from build123d import *

# Parameters (mm, degrees)
SKETCH1_R           = 45
SKETCH1_R_2         = 15
SKETCH1_R_3         = 2.5
BOSS_EXTRUDE1_DEPTH = 3
SKETCH2_R           = 4
SKETCH2_R_2         = 2.5
BOSS_EXTRUDE2_DEPTH = 1
FILLET1_R           = 0.25


with BuildPart() as part:
    # Sketch1 → Boss-Extrude1 (new body)
    with BuildSketch(Plane(origin=(0, 0, 0), x_dir=(1, 0, 0), z_dir=(0, 1, 0))):
        with Locations(Location((0, 0, 0), (0, 0, 270))):
            Circle(SKETCH1_R)
        with Locations(Location((0, 0, 0), (0, 0, 270))):
            Circle(SKETCH1_R_2, mode=Mode.SUBTRACT)
        with Locations(Location((0, 25, 0), (0, 0, 270))):
            Circle(SKETCH1_R_3, mode=Mode.SUBTRACT)
        with Locations(Location((25, 0, 0), (0, 0, 270))):
            Circle(SKETCH1_R_3, mode=Mode.SUBTRACT)
        with Locations(Location((0, -25, 0), (0, 0, 270))):
            Circle(SKETCH1_R_3, mode=Mode.SUBTRACT)
        with Locations(Location((-25, 0, 0), (0, 0, 270))):
            Circle(SKETCH1_R_3, mode=Mode.SUBTRACT)
    extrude(amount=BOSS_EXTRUDE1_DEPTH)

    # Sketch2 → Boss-Extrude2 (add)
    # profile 1 of 4: a face of its own
    with BuildSketch(Plane(origin=(0, 3, 0), x_dir=(1, 0, 0), z_dir=(0, 1, 0))):
        with Locations(Location((25, 0, 0), (0, 0, 270))):
            Circle(SKETCH2_R)
        with Locations(Location((25, 0, 0), (0, 0, 270))):
            Circle(SKETCH2_R_2, mode=Mode.SUBTRACT)
    # profile 2 of 4: a face of its own
    with BuildSketch(Plane(origin=(0, 3, 0), x_dir=(1, 0, 0), z_dir=(0, 1, 0))):
        with Locations(Location((0, 25, 0), (0, 0, 270))):
            Circle(SKETCH2_R)
        with Locations(Location((0, 25, 0), (0, 0, 270))):
            Circle(SKETCH2_R_2, mode=Mode.SUBTRACT)
    # profile 3 of 4: a face of its own
    with BuildSketch(Plane(origin=(0, 3, 0), x_dir=(1, 0, 0), z_dir=(0, 1, 0))):
        with Locations(Location((0, -25, 0), (0, 0, 270))):
            Circle(SKETCH2_R)
        with Locations(Location((0, -25, 0), (0, 0, 270))):
            Circle(SKETCH2_R_2, mode=Mode.SUBTRACT)
    # profile 4 of 4: a face of its own
    with BuildSketch(Plane(origin=(0, 3, 0), x_dir=(1, 0, 0), z_dir=(0, 1, 0))):
        with Locations(Location((-25, 0, 0), (0, 0, 270))):
            Circle(SKETCH2_R)
        with Locations(Location((-25, 0, 0), (0, 0, 270))):
            Circle(SKETCH2_R_2, mode=Mode.SUBTRACT)
    extrude(amount=BOSS_EXTRUDE2_DEPTH)

    # Fillet1
    fillet1_edges = [part.edges().sort_by_distance(p)[0] for p in [
        (-25, 4, -4),
        (0, 4, 21),
        (25, 4, -4),
        (0, 4, -29),
    ]]
    fillet(fillet1_edges, radius=FILLET1_R)


solid = part.part
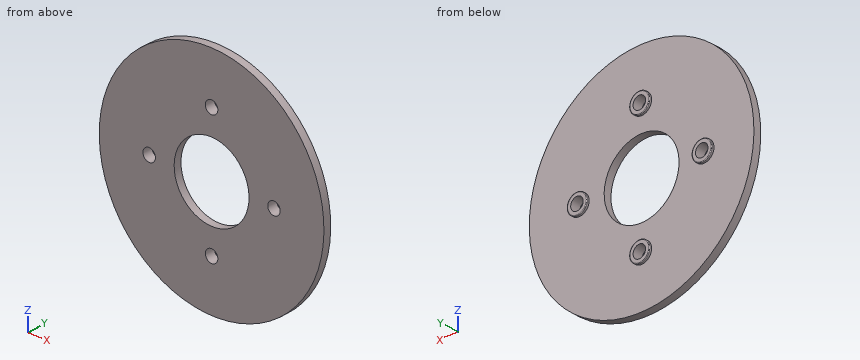
CAD build for the part. Positions are in the model's coordinates, mm. Give positions to 0.01 mm unless a question says otherwise; leave off trailing zeros. Write each loop counter-clockwise with the first axis right and the second up, starting at its lowest first coordinate (ties: lowest second). Pieces come first, ordered by that corner, then holes. Notation, with made-up numbers: (62.5, 50) - (95.5, 50) arc R14 cw to (95.5, 61) - close; hole circle Ø7 at (70.5, 24). An arc over 180 degrees is marked (long way). Answer as CSV lines item,"result".
Q1. Band-saw the part on B-B (z = 0). Give the cut face in (x, y).
Result set:
outline,"(-45, 0) - (-27.5, 0) - (-27.5, 4) - (-28.75, 4) arc R0.25 ccw to (-29, 3.75) - (-29, 3) - (-45, 3) - close; (-22.5, 0) - (-15, 0) - (-15, 3) - (-21, 3) - (-21, 3.75) arc R0.25 ccw to (-21.25, 4) - (-22.5, 4) - close; (15, 0) - (22.5, 0) - (22.5, 4) - (21.25, 4) arc R0.25 ccw to (21, 3.75) - (21, 3) - (15, 3) - close; (27.5, 0) - (45, 0) - (45, 3) - (29, 3) - (29, 3.75) arc R0.25 ccw to (28.75, 4) - (27.5, 4) - close"
Q2. Band-saw the part on C-C (y = 1.75). Give the cut face in (x, z), and give its area (3 significant figures).
Result set:
outline,"circle Ø90 at (0, 0); hole circle Ø5 at (-25, 0); hole circle Ø30 at (0, 0); hole circle Ø5 at (0, -25); hole circle Ø5 at (0, 25); hole circle Ø5 at (25, 0)"
area,"5,580 mm²"
Q3. Band-saw the part on A-A (x = 0). Give the cut face in (y, z), and give its area (3 significant figures).
Result set:
outline,"(0, -45) - (3, -45) - (3, -29) - (3.75, -29) arc R0.25 ccw to (4, -28.75) - (4, -27.5) - (0, -27.5) - close; (0, -22.5) - (4, -22.5) - (4, -21.25) arc R0.25 ccw to (3.75, -21) - (3, -21) - (3, -15) - (0, -15) - close; (0, 15) - (3, 15) - (3, 21) - (3.75, 21) arc R0.25 ccw to (4, 21.25) - (4, 22.5) - (0, 22.5) - close; (0, 27.5) - (4, 27.5) - (4, 28.75) arc R0.25 ccw to (3.75, 29) - (3, 29) - (3, 45) - (0, 45) - close"
area,"156 mm²"
Q4. Band-saw the part on D-D (z = -25). Give the cut face in (x, y).
Result set:
outline,"(-37.42, 0) - (-2.5, 0) - (-2.5, 4) - (-3.75, 4) arc R0.25 ccw to (-4, 3.75) - (-4, 3) - (-37.42, 3) - close; (2.5, 0) - (37.42, 0) - (37.42, 3) - (4, 3) - (4, 3.75) arc R0.25 ccw to (3.75, 4) - (2.5, 4) - close"
Q5. Drill centre lines: line 1 (X direction, y = 2.2, z = 0); line 2 (Z direction, x = -2, y = 0.7); line 3 (Y direction, x = 32.5, z = 24). Where is each one in solid material? Low to high. Write a range as from..to.
Result set:
line 1,"-45..-27.5, -22.5..-15, 15..22.5, 27.5..45"
line 2,"-44.96..-26.5, -23.5..-14.87, 14.87..23.5, 26.5..44.96"
line 3,"0..3"
Q6. Flat gauge pins, fed straight in: pin 1 Ø1.5 at (y, z) = (2.5, 18.5) entering from +X; pin 2 Ø4 at (x, z) = (31.5, -10) entering from +Y; pin 3 Ø2 at (y, z) = (3, 5.5) entering from -X. Where does each tip first touch, or does it go through?
Result set:
pin 1,"x = 41.35"
pin 2,"y = 3"
pin 3,"x = -44.77"
